from build123d import *

# Parameters (mm, degrees)
SKETCH1_R           = 2.5
BOSS_EXTRUDE1_DEPTH = 5
SKETCH2_R           = 1
CUT_EXTRUDE1_DEPTH  = 101.623058987
SKETCH3_R           = 5
BEARINGBORE_DEPTH   = 101.623058987


with BuildPart() as part:
    # Sketch1 → Boss-Extrude1 (new body)
    with BuildSketch(Plane(origin=(0, 0, 0), x_dir=(1, 0, 0), z_dir=(0, 1, 0))):
        with BuildLine():
            Line((-10, -90), (-10, 90))
            ThreePointArc((-10, 90), (0, 100), (10, 90))
            Line((10, 90), (10, -90))
            ThreePointArc((10, -90), (0, -100), (-10, -90))
        make_face()
        with Locations(Location((0, 90, 0), (0, 0, 270))):
            Circle(SKETCH1_R, mode=Mode.SUBTRACT)
    extrude(amount=BOSS_EXTRUDE1_DEPTH)

    # Sketch2 → Cut-Extrude1 (cut, through all)
    with BuildSketch(Plane.XZ):
        with Locations(Location((0, -71.209904471, 0), (0, 0, 270))):
            Circle(SKETCH2_R)
    extrude(amount=-CUT_EXTRUDE1_DEPTH, mode=Mode.SUBTRACT)

    # Sketch3 → BearingBore (cut, through all)
    with BuildSketch(Plane(origin=(0, 5, 0), x_dir=(1, 0, 0), z_dir=(0, 1, 0))):
        with Locations(Location((0, -90, 0), (0, 0, 270))):
            Circle(SKETCH3_R)
    extrude(amount=-BEARINGBORE_DEPTH, mode=Mode.SUBTRACT)


solid = part.part
Check sheet for the modelled part. Datum: model origin and axes. Units: mm. Coordinates: 2 decimals unless noted, no trailing zeros. Write each loop counter-clockwise with the first axis right and the second up, starting at its lowest first coordinate (ties: lowest second). Pieces come first, ordered by that corner, then holes. Notation, with made-up numbers: M 29,-25.75 L 72,-25.75 A29 ccw 72,2.25 Z; hole C 88.5,2 d3. An arc over 180 degrees is marked long. Answer as CSV lines item,"result".
Q1. Go/stop test with flat-tipped pins: pin 1 (2 mm diameter, centred on x = -3, y = 1, fed in from +Z); pin 2 (6 mm diameter, centred on x = 0, z = -90, fed in from +Y); pin 3 (3 mm diameter, centred on x = 3.5, y = 0.5, fed in from -Z). Record where each tip stops, or that it passes through.
Check result:
pin 1,"z = 99.8"
pin 2,"y = 5"
pin 3,"z = -99.8"
Q2. Material ranges on probe 1 along X at (y, z) = (3.4, 90); probe 2 along X at (y, z) = (4.4, -90); probe 3 along Z at (x, y) = (-4, 1.95), recorded low to high. Write a range as from..to.
Check result:
probe 1,"-10..-5, 5..10"
probe 2,"-10..-2.5, 2.5..10"
probe 3,"-99.17..87, 93..99.17"
Q3. Cross-section at B-B (x = -8). Record the boundary of the cut face in (y, z).
Check result:
outline,"M 0,-96 L 5,-96 L 5,96 L 0,96 Z"
Q4. Cross-section at A-A (y = 2). Record the boundary of the cut face in (x, z), then the cut area to 3 significant figures.
Check result:
outline,"M -10,-90 A10 ccw 10,-90 L 10,90 A10 ccw -10,90 Z; hole C 0,90 d10; hole C 0,-90 d5; hole C 0,-71.21 d2"
area,"3,810 mm^2"
Q5. Mould release check, pull along Z, two halves, no side actions. Record for faces 1 (the face through (10, 2, -1)), 2 (the face through (0.1, 2.5, -92.5)), 3 (the face through (0, 2, 100)): released by +Z, released by -Z, zero draft, split by the parting line, or undercut.
Check result:
face 1,"zero draft"
face 2,"undercut"
face 3,"released by +Z"
Q6. Cross-section at C-C (x = 7). Record the boundary of the cut face in (y, z), then the cut area to 3 significant figures.
Check result:
outline,"M 0,-97.14 L 5,-97.14 L 5,97.14 L 0,97.14 Z"
area,"971 mm^2"
